Input: part model. Units: mm. Frame: model coordinates. Face numbers are marked on the shaded views. A direction names the side the tool comes from. Round coordinates to 2 decimals unless told otherwise and drop trailing zeros. Loops run counter-clockwise (first coordinate to the right, second up) from the corner with the lowest first, then second, coordinate; pieces in that order, holes last. Notation, with made-up numbers: (29.25, 83) -> (53.25, 83) arc R33 cw to (53.25, 116) -> close; hole circle Ø9 at (38.25, 4.5). An arc over 180 degrees is marked (long way). Answer as a JSON object with one key per item and string values. Group by question number.
Item 1: Material intervals for line 1 (Y direction, x = -25.4, z = 6.25) (3 decimals); line 2 (X direction, y = -44, z = 23); line 3 (X direction, y = -25.4, z = 11.5) (3 decimals), sorted ascending. Write a range as [from, to].
Item 2: Draft query along Y for the marked faces 3, 4 and 5. Return one class per face: released by +Y, released by -Y, zero draft, split by the parting line, or undercut.
Item 3: Section query C-C on z = 4.75. Return loops of the section in (x, y) (3 decimals), and give its area (3 significant figures).
Item 4: Section query A-A on y = -25.4. Return loops of the section in (x, z) (3 decimals).
Item 5: Pin query (flat end, axial travel): pin 1 (5 mm diameter, centred on x = -20, y = -26, fed in from -Z); pin 2 (6.5 mm diameter, centred on x = 9, y = -45, fed in from +Z). Return the tip coordinate at first contact, or that it passes through.
Item 6: Section query D-D on y = -41. Return loops of the section in (x, z), and give its area (3 significant figures).
Item 7: Section query B-B on x = -25.4. Return loops of the section in (y, z) (3 decimals), and give its area (3 significant figures).
Item 8: Set-up query: the marked faces 1 and 2. Return all of +Z, -Z, +X, -X, +Y, -Y with unobstructed straight access to the full face (end or side cutting, diameter ignored); none if empty.
from build123d import *

# Parameters (mm, degrees)
F1_DEPTH = 76.2
F2_R     = 9.525
F3_DEPTH = 76.2


with BuildPart() as f1:
    # F0 (on Front) → F1 (new body)
    with BuildSketch(Plane.XZ):
        Polygon((-50.8, 0), (25.4, 0), (25.4, 25.4), (12.7, 25.4), (12.7, 19.05), (0, 19.05), (0, 25.4), (-50.8, 25.4), align=None)
    extrude(amount=F1_DEPTH)

    # F2 (on Top) → F3 (cut)
    with BuildSketch(Plane.XY):
        with Locations((-25.4, -25.4)):
            Circle(F2_R)
    extrude(amount=F3_DEPTH, mode=Mode.SUBTRACT)


solid = f1.part
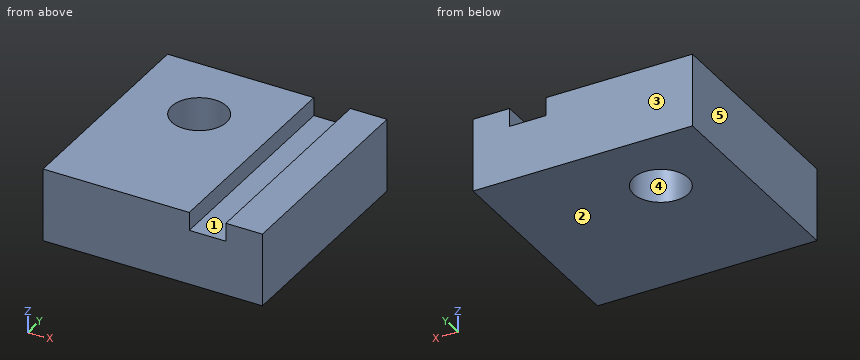
Solved:
{
 "1": {"line 1": "[-76.2, -34.925], [-15.875, 0]", "line 2": "[-50.8, 0], [12.7, 25.4]", "line 3": "[-50.8, -34.925], [-15.875, 25.4]"},
 "2": {"face 3": "released by +Y", "face 4": "undercut", "face 5": "zero draft"},
 "3": {"outline": "(-50.8, -76.2) -> (25.4, -76.2) -> (25.4, 0) -> (-50.8, 0) -> close; hole circle Ø19.05 at (-25.4, -25.4)", "area": "5,520 mm²"},
 "4": {"outline": "(-50.8, 0) -> (-34.925, 0) -> (-34.925, 25.4) -> (-50.8, 25.4) -> close; (-15.875, 0) -> (25.4, 0) -> (25.4, 25.4) -> (12.7, 25.4) -> (12.7, 19.05) -> (0, 19.05) -> (0, 25.4) -> (-15.875, 25.4) -> close"},
 "5": {"pin 1": "through", "pin 2": "z = 19.05"},
 "6": {"outline": "(-50.8, 0) -> (25.4, 0) -> (25.4, 25.4) -> (12.7, 25.4) -> (12.7, 19.05) -> (0, 19.05) -> (0, 25.4) -> (-50.8, 25.4) -> close", "area": "1,850 mm²"},
 "7": {"outline": "(-76.2, 0) -> (-34.925, 0) -> (-34.925, 25.4) -> (-76.2, 25.4) -> close; (-15.875, 0) -> (0, 0) -> (0, 25.4) -> (-15.875, 25.4) -> close", "area": "1,450 mm²"},
 "8": {"face 1": "+Z, +Y, -Y", "face 2": "-Z, +X, -X, +Y, -Y"}
}
